Can you work these out from the model? Positions are in its coordinate system, mm. Face numbers are marked on the shaded views. Coordinates: 2 decimals unless noted, no trailing zeros. Write each loop counter-clockwise with the first axis right and the second up, starting at its lowest first coordinate (ties: lowest second). Pieces come first, ordered by that corner, then holes. Notation, with made-up numbers: M 54,23 L 78,23 A14 cw 78,37 Z; hole C 41,17.25 d3. An arc over 180 degrees is marked long. Answer as a JSON object with one key per item and string values. Group by question number.
from build123d import *

# Parameters (mm, degrees)
F0_W     = 140.431046
F0_H     = 109.784484
F1_DEPTH = 25
F2_R     = 26.666566
F3_DEPTH = 40
F5_DEPTH = 128


with BuildPart() as f1:
    # F0 (on Top) → F1 (new body)
    with BuildSketch(Plane.XY):
        Rectangle(F0_W, F0_H)
    extrude(amount=-F1_DEPTH)

    # F2 (on face) → F3 (join)
    with BuildSketch(Plane.XY):
        Circle(F2_R)
    extrude(amount=F3_DEPTH)

    # F4 (on face) → F5 (cut)
    with BuildSketch(Plane.XZ.offset(54.892242)):
        Polygon((-26.627764, 40.126272), (26.686043, 0), (26.686043, 40.126272), align=None)
    extrude(amount=-F5_DEPTH, mode=Mode.SUBTRACT)


solid = f1.part
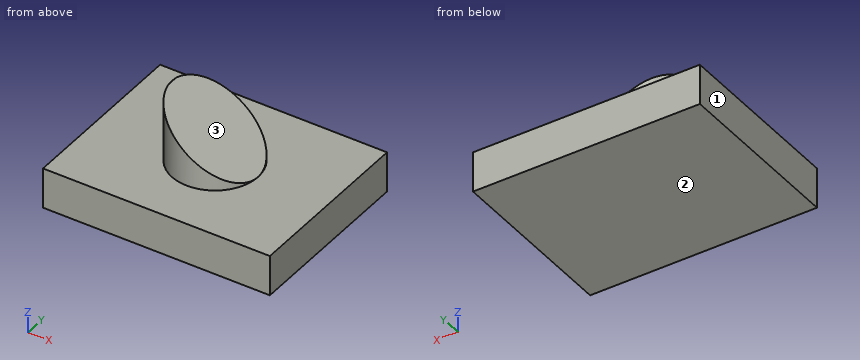
Q1. We'd pull the mould along X, two halves only. Please class the marked faces 1, 2 and 3: pulls with the +X half, pulls with the -X half, needs draft (parallel to the pull), parting line crosses it, or undercut.
Q2. If we section it at B-B on x = 0: List the corners of the cut face in (y, z) for me.
Q3. Will these pins go through, and if not, where does the flat tip stop? pin 1 (1.5 mm diameter, centred on y = 19.5, z = 21, fed in from +X); pin 2 (10 mm diameter, centred on y = -13.5, z = 32.5, fed in from +X); pin 3 (4 mm diameter, centred on y = 17, z = 8, fed in from -X).
Q4. If we section it at C-C on z = 13.5: List the corners of the cut face in (x, y) for me.
Q5. If we section it at D-D on y = -43: List the corners of the cut face in (x, z) for me, and give its area (3 significant figures).
Q6. Please list where these lines run through material, in increasing order: L1, parallel to Z at x = 53, y = 27.5; L2, parallel to X at y = 12, z = 16.5; L3, parallel to X at y = 13.5, z = 8.5.
Reply:
{
 "1": {"face 1": "pulls with the -X half", "face 2": "needs draft", "face 3": "pulls with the +X half"},
 "2": {"outline": "M -54.89,-25 L 54.89,-25 L 54.89,0 L 26.67,0 L 26.67,20.09 L -26.67,20.09 L -26.67,0 L -54.89,0 Z"},
 "3": {"pin 1": "x = -0.22", "pin 2": "x = -9.85", "pin 3": "x = -22.05"},
 "4": {"outline": "M 8.75,-25.19 L 8.75,25.19 A26.67 ccw long Z"},
 "5": {"outline": "M -70.22,-25 L 70.22,-25 L 70.22,0 L -70.22,0 Z", "area": "3,510 mm^2"},
 "6": {"L1": "-25 to 0", "L2": "-23.81 to 4.76", "L3": "-23 to 15.39"}
}
